from build123d import *

# Parameters (mm, degrees)
SKETCH_1_R          = 2.175
EXTRUDE_4_DEPTH     = 6
SKETCH_1_3_R        = 2.175
CUT_EXTRUDE_3_DEPTH = 4.5
SKETCH_8_R          = 2.55
EXTRUDE_5_DEPTH     = 11
FILLET_1_R          = 2
CUT_EXTRUDE_START   = -5
SKETCH_8_2_R        = 2.55
CUT_EXTRUDE_4_DEPTH = 5
CHAMFER_1_SIZE      = 1


with BuildPart() as part:
    # 草图1 → 凸台-拉伸4 (new body)
    # profile 1 of 6: a face of its own
    with BuildSketch(Plane(origin=(0, 0, 0), x_dir=(1, 0, 0), z_dir=(0, 1, 0))):
        with BuildLine():
            Line((-13.5, 16.5), (13.5, 16.5))
            ThreePointArc((13.5, 16.5), (15.621320344, 15.621320344), (16.5, 13.5))
            Line((16.5, 13.5), (16.5, -13.5))
            ThreePointArc((16.5, -13.5), (15.621320344, -15.621320344), (13.5, -16.5))
            Line((13.5, -16.5), (-13.5, -16.5))
            ThreePointArc((-13.5, -16.5), (-15.621320344, -15.621320344), (-16.5, -13.5))
            Line((-16.5, -13.5), (-16.5, 13.5))
            ThreePointArc((-16.5, 13.5), (-15.621320344, 15.621320344), (-13.5, 16.5))
        make_face()
        with Locations((-10.5, 10.5)):
            Circle(SKETCH_1_R, mode=Mode.SUBTRACT)
        with Locations((10.5, 10.5)):
            Circle(SKETCH_1_R, mode=Mode.SUBTRACT)
        with Locations((10.5, -10.5)):
            Circle(SKETCH_1_R, mode=Mode.SUBTRACT)
        with Locations((-10.5, -10.5)):
            Circle(SKETCH_1_R, mode=Mode.SUBTRACT)
        Circle(SKETCH_1_R, mode=Mode.SUBTRACT)
    # profile 2 of 6: a face of its own
    with BuildSketch(Plane(origin=(0, 0, 0), x_dir=(1, 0, 0), z_dir=(0, 1, 0))):
        with Locations((10.5, -10.5)):
            Circle(SKETCH_1_R)
    # profile 3 of 6: a face of its own
    with BuildSketch(Plane(origin=(0, 0, 0), x_dir=(1, 0, 0), z_dir=(0, 1, 0))):
        with Locations((10.5, 10.5)):
            Circle(SKETCH_1_R)
    # profile 4 of 6: a face of its own
    with BuildSketch(Plane(origin=(0, 0, 0), x_dir=(1, 0, 0), z_dir=(0, 1, 0))):
        with Locations((-10.5, 10.5)):
            Circle(SKETCH_1_R)
    # profile 5 of 6: a face of its own
    with BuildSketch(Plane(origin=(0, 0, 0), x_dir=(1, 0, 0), z_dir=(0, 1, 0))):
        Circle(SKETCH_1_R)
    # profile 6 of 6: a face of its own
    with BuildSketch(Plane(origin=(0, 0, 0), x_dir=(1, 0, 0), z_dir=(0, 1, 0))):
        with Locations((-10.5, -10.5)):
            Circle(SKETCH_1_R)
    extrude(amount=EXTRUDE_4_DEPTH)

    # 草图1<3> → 切除-拉伸3 (cut)
    with BuildSketch(Plane(origin=(0, 0, 0), x_dir=(1, 0, 0), z_dir=(0, 1, 0))):
        with Locations(Location((10.5, -10.5, 0), (0, 0, 270))):
            Circle(SKETCH_1_3_R)
        with Locations(Location((10.5, 10.5, 0), (0, 0, 270))):
            Circle(SKETCH_1_3_R)
        with Locations(Location((-10.5, 10.5, 0), (0, 0, 270))):
            Circle(SKETCH_1_3_R)
        with Locations(Location((-10.5, -10.5, 0), (0, 0, 270))):
            Circle(SKETCH_1_3_R)
        with Locations(Location((0, 0, 0), (0, 0, 270))):
            Circle(SKETCH_1_3_R)
    extrude(amount=CUT_EXTRUDE_3_DEPTH, mode=Mode.SUBTRACT)

    # 草图8 → 凸台-拉伸5 (add)
    with BuildSketch(Plane(origin=(0, 6, 0), x_dir=(1, 0, 0), z_dir=(0, 1, 0))):
        with BuildLine():
            Line((-9.5, 12.5), (9.5, 12.5))
            ThreePointArc((9.5, 12.5), (11.621320344, 11.621320344), (12.5, 9.5))
            Line((12.5, 9.5), (12.5, -9.5))
            ThreePointArc((12.5, -9.5), (11.621320344, -11.621320344), (9.5, -12.5))
            Line((9.5, -12.5), (-9.5, -12.5))
            ThreePointArc((-9.5, -12.5), (-11.621320344, -11.621320344), (-12.5, -9.5))
            Line((-12.5, -9.5), (-12.5, 9.5))
            ThreePointArc((-12.5, 9.5), (-11.621320344, 11.621320344), (-9.5, 12.5))
        make_face()
        with Locations(Location((-6.25, 6.25, 0), (0, 0, 270))):
            Circle(SKETCH_8_R, mode=Mode.SUBTRACT)
        with Locations(Location((6.25, 6.25, 0), (0, 0, 270))):
            Circle(SKETCH_8_R, mode=Mode.SUBTRACT)
        with Locations(Location((-6.25, -6.25, 0), (0, 0, 270))):
            Circle(SKETCH_8_R, mode=Mode.SUBTRACT)
        with Locations(Location((6.25, -6.25, 0), (0, 0, 270))):
            Circle(SKETCH_8_R, mode=Mode.SUBTRACT)
    extrude(amount=EXTRUDE_5_DEPTH)

    # 圆角1
    fillet_1_edges = [part.edges().sort_by_distance(p)[0] for p in [
        (11.621320344, 6, 11.621320344),
        (12.5, 6, 0),
        (11.621320344, 6, -11.621320344),
        (0, 6, -12.5),
        (-11.621320344, 6, -11.621320344),
        (-12.5, 6, 0),
        (-11.621320344, 6, 11.621320344),
        (0, 6, 12.5),
    ]]
    fillet(fillet_1_edges, radius=FILLET_1_R)

    # 草图8<2> → 切除-拉伸4 (cut)
    with BuildSketch(Plane(origin=(0, 6, 0), x_dir=(1, 0, 0), z_dir=(0, 1, 0)).offset(CUT_EXTRUDE_START)):
        with Locations(Location((-6.25, 6.25, 0), (0, 0, 270))):
            Circle(SKETCH_8_2_R)
        with Locations(Location((6.25, 6.25, 0), (0, 0, 270))):
            Circle(SKETCH_8_2_R)
        with Locations(Location((6.25, -6.25, 0), (0, 0, 270))):
            Circle(SKETCH_8_2_R)
        with Locations(Location((-6.25, -6.25, 0), (0, 0, 270))):
            Circle(SKETCH_8_2_R)
    extrude(amount=CUT_EXTRUDE_4_DEPTH, mode=Mode.SUBTRACT)

    # 倒角1
    chamfer_1_edges = [part.edges().sort_by_distance(p)[0] for p in [
        (-16.5, 6, 0),
        (-15.621320344, 6, 15.621320344),
        (0, 6, 16.5),
        (15.621320344, 6, 15.621320344),
        (16.5, 6, 0),
        (15.621320344, 6, -15.621320344),
        (0, 6, -16.5),
        (-15.621320344, 6, -15.621320344),
    ]]
    chamfer(chamfer_1_edges, length=CHAMFER_1_SIZE)


solid = part.part
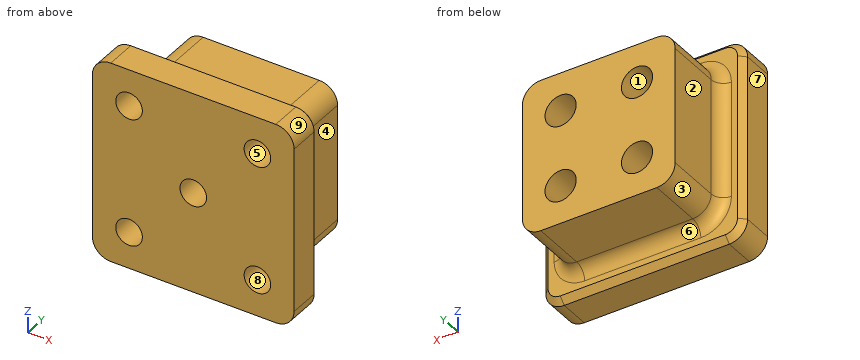
Check sheet for the modelled part. Datum: model origin and axes. Units: mm. Face numbers are marked on the shaded views. A direction names the side the tool comes from. Round coordinates to 2 decimals unless told otherwise and drop trailing zeros. Order: outer loops, then holes, each group sorted by start corner. A loop starts at its lowest first (then second) coordinate and runs counter-clockwise, first axis right, second up.
(1) Draft check along X on the marked faces 6, 7, 8 and 9. Enter one of: pulls with the +X half, pulls with the -X half, needs draft (parallel to the pull), parting line crosses it, or undercut.
(2) Scan lines: probe 1 along X at (y, z) = (3.2, -10.5) (3 decimals); probe 2 along Z at (x, y) = (5, 10); probe 3 along X at (y, z) = (12.75, 6.25). Record each from-to range of solid material in increasing order.
(3) Cross-section at B-B, the plane x = 0. Enter the section's corners in (y, z) (3 decimals).
(4) Cross-section at D-D, the plane x = -6.25. Enter the section's corners in (y, z).
(5) Cross-section at C-C, the plane z = -6.25. Enter the section's corners in (x, y).
(6) Go/stop test with flat-tipped pins: P1, Ø2, axis at x = 0.5, z = 1, coming from the -Y side; P2, Ø3.5, axis at x = -11, z = 11, coming from the -Y side; P3, Ø3, axis at y = 14.5, z = 4, coming from the +X side; P4, Ø4.5, axis at x = 0.5, y = 12.5, coming from the -Z side. Record where each tip stops, or that it passes through.
(7) Cross-section at A-A, the plane y = 15.25. Enter the section's corners in (x, z).
(8) Access from +Z, -Z, +X, -X, +Y, -Y to the whole of each face (thin tool, end or side, straight path). Record for the marked faces 1, 2, 3, 4 and 5.
Check sheet entries:
1. face 6: needs draft
1. face 7: pulls with the -X half
1. face 8: undercut
1. face 9: pulls with the +X half
2. probe 1: x = -16.5 to -12.675, -8.325 to 8.325, 12.675 to 16.5
2. probe 2: z = -12.5 to -8.47, -4.03 to 4.03, 8.47 to 12.5
2. probe 3: x = -12.5 to -8.8, -3.7 to 3.7, 8.8 to 12.5
3. outline: (0, -16.5) - (5, -16.5) - (6, -15.5) - (6, -14.5) arc R2 cw to (8, -12.5) - (17, -12.5) - (17, 12.5) - (8, 12.5) arc R2 cw to (6, 14.5) - (6, 15.5) - (5, 16.5) - (0, 16.5) - (0, 2.175) - (4.5, 2.175) - (4.5, -2.175) - (0, -2.175) - close
4. outline: (0, -16.5) - (5, -16.5) - (6, -15.5) - (6, -14.5) arc R2 cw to (8, -12.5) - (17, -12.5) - (17, -8.8) - (1, -8.8) - (1, -3.7) - (17, -3.7) - (17, 3.7) - (1, 3.7) - (1, 8.8) - (17, 8.8) - (17, 12.5) - (8, 12.5) arc R2 cw to (6, 14.5) - (6, 15.5) - (5, 16.5) - (0, 16.5) - close
5. outline: (-16.5, 0) - (16.5, 0) - (16.5, 5) - (15.5, 6) - (14.5, 6) arc R2 cw to (12.5, 8) - (12.5, 17) - (8.8, 17) - (8.8, 1) - (3.7, 1) - (3.7, 17) - (-3.7, 17) - (-3.7, 1) - (-8.8, 1) - (-8.8, 17) - (-12.5, 17) - (-12.5, 8) arc R2 cw to (-14.5, 6) - (-15.5, 6) - (-16.5, 5) - close
6. P1: stops at y = 4.5
6. P2: stops at y = 0
6. P3: stops at x = 12.5
6. P4: stops at z = -12.5
7. outline: (-12.5, -9.5) arc R3 ccw to (-9.5, -12.5) - (9.5, -12.5) arc R3 ccw to (12.5, -9.5) - (12.5, 9.5) arc R3 ccw to (9.5, 12.5) - (-9.5, 12.5) arc R3 ccw to (-12.5, 9.5) - close; hole circle Ø5.1 at (-6.25, -6.25); hole circle Ø5.1 at (-6.25, 6.25); hole circle Ø5.1 at (6.25, -6.25); hole circle Ø5.1 at (6.25, 6.25)
8. face 1: +Y
8. face 2: +Z, -Z, -X, +Y
8. face 3: -Z, -X, +Y
8. face 4: +Z, -Z, +X, +Y
8. face 5: -Y
